Geometry: final body of the model. Coordinates: model frame, mm. Coordinates: 2 decimals unless noted, no trailing zeros. Write each loop counter-clockwise with the first axis right and the second up, starting at its lowest first coordinate (ties: lowest second). Pieces come first, ordered by that corner, then holes.
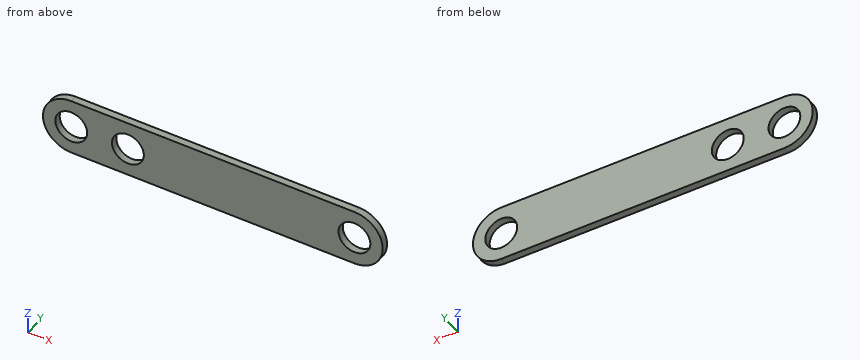
Autodesk Inventor part; units mm, degrees
ref_plane "YZ Plane" through (0, 0, 0) normal (1, 0, 0) x (0, 1, 0)
ref_plane "XZ Plane" through (0, 0, 0) normal (0, 1, 0) x (-1, 0, 0)
ref_plane "XY Plane" through (0, 0, 0) normal (0, 0, 1) x (1, 0, 0)
sketch "Sketch1" plane through (0, 0, 0) normal (0, 1, 0) x (-1, 0, 0)
  line L0 (0, 0) -> (-203.2, 0)
  line L1 (0, 25.4) -> (-76.2, 25.4) construction
  line L2 (-203.2, 25.4) -> (-127, 25.4) construction
  line L3 (-127, 25.4) -> (-330.2, 25.4)
  line L4 (0, 0) -> (-203.2, 0)
  line L5 (-203.2, 50.8) -> (0, 50.8)
  line L6 (-203.2, 0) -> (-330.2, 0)
  line L7 (-203.2, 50.8) -> (-330.2, 50.8)
  arc A0 (-330.2, 50.8) -> (-330.2, 0) centre (-330.2, 25.4) ccw
  arc A1 (0, 0) -> (0, 50.8) centre (0, 25.4) ccw
  arc A2 (-76.2, 0) -> (-76.2, 50.8) centre (-76.2, 25.4) ccw
  circle A3 centre (-330.2, 25.4) radius 14.2875
  circle A4 centre (-127, 25.4) radius 14.2875
  circle A5 centre (-76.2, 25.4) radius 14.2875
  point P0 (-331.4575, 38.0376)
  point P1 (-331.4575, 12.7624)
  point P2 (-76.2, 0)
  dimension "d2" = 76.2
  dimension "d3" = 76.2
  dimension "d8" = 203.2
  dimension "d12" = 50.8
  dimension "d17" = 28.575
  dimension "d18" = 28.575
  dimension "d19" = 28.575
extrude "Extrusion1" add sketch "Sketch1" along normal blind 6.35 contours L0 L6 A0 L7 L5 A2
properties part number "4-bar intake block"
Item 1: Section A-A, the plane z = 25.4. Output: boundary loops of the cut face in (x, y), plus the area to 3 significant figures.
Derived:
outline: (50.8, 0) - (61.91, 0) - (61.91, 6.35) - (50.8, 6.35) - close; (90.49, 0) - (112.71, 0) - (112.71, 6.35) - (90.49, 6.35) - close; (141.29, 0) - (315.91, 0) - (315.91, 6.35) - (141.29, 6.35) - close; (344.49, 0) - (355.6, 0) - (355.6, 6.35) - (344.49, 6.35) - close
area: 1,390 mm2
Item 2: Section B-B, the plane y = 3.5. Output: boundary loops of the cut face in (x, z) (1 decimal).
Derived:
outline: (76.2, 0) - (330.2, 0) arc R25.4 ccw to (330.2, 50.8) - (76.2, 50.8) arc R25.4 ccw to start; hole circle Ø28.6 at (76.2, 25.4); hole circle Ø28.6 at (127, 25.4); hole circle Ø28.6 at (330.2, 25.4)
Item 3: Section D-D, the plane z = 14.5. Output: boundary loops of the cut face in (x, y), plus the area to 3 significant figures.
Derived:
outline: (53.26, 0) - (66.96, 0) - (66.96, 6.35) - (53.26, 6.35) - close; (85.44, 0) - (117.76, 0) - (117.76, 6.35) - (85.44, 6.35) - close; (136.24, 0) - (320.96, 0) - (320.96, 6.35) - (136.24, 6.35) - close; (339.44, 0) - (353.14, 0) - (353.14, 6.35) - (339.44, 6.35) - close
area: 1,550 mm2
Item 4: Pin query (flat end, axial travel): pin 1 (3 mm diameter, centred on y = 4, z = 45.5, fed in from -X); pin 2 (8 mm diameter, centred on x = 138, z = 28, fed in from -Y); pin 3 (3 mm diameter, centred on y = 3.5, z = 29, fed in from -X). Return the tip coordinate at first contact, or that it passes through.
Derived:
pin 1: stops at x = 58.9
pin 2: stops at y = 0
pin 3: stops at x = 50.89
Item 5: Section C-C, the plane x = 127. Output: boundary loops of the cut face in (y, z).
Derived:
outline: (0, 0) - (6.35, 0) - (6.35, 11.11) - (0, 11.11) - close; (0, 39.69) - (6.35, 39.69) - (6.35, 50.8) - (0, 50.8) - close
Item 6: Material intervals for probe 1 along X at (y, z) = (4.75, 31.5); probe 2 along Z at (x, y) = (76.2, 3.5); probe 3 along X at (y, z) = (5.5, 32.5), sorted ascending.
Derived:
probe 1: x = 51.54 to 63.28, 89.12 to 114.08, 139.92 to 317.28, 343.12 to 354.86
probe 2: z = 0 to 11.11, 39.69 to 50.8
probe 3: x = 51.81 to 63.8, 88.6 to 114.6, 139.4 to 317.8, 342.6 to 354.59
